Read the model definition and answer for the solid it produces. Units are mm, in the model's axes. Face numbers are marked on the shaded views. A direction names the side the tool comes from. Coordinates: 2 decimals unless noted, no trailing zeros. Loops run counter-clockwise (first coordinate to the right, second up) from the corner with the lowest first, then second, coordinate; pieces in that order, holes last. Notation, with made-up numbers: M 31,3.5 L 61,3.5 A17 cw 61,8.5 Z; hole C 43.5,34 d1. An arc over 180 degrees is marked long. One line per item, written item: value. Start each with the question number.
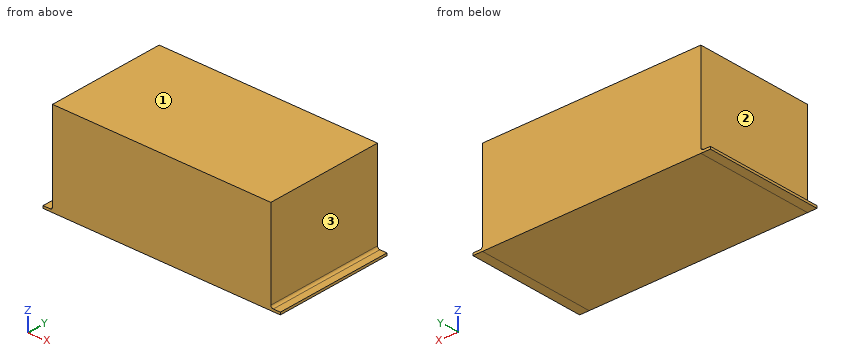
```python
from build123d import *

# Parameters (mm, degrees)
IZIM1_W                     = 920
IZIM1_H                     = 500
Y_KSEKLIK_EKSTR_ZYON1_DEPTH = 380
BO_ALTMA1_T                 = -0.6
IZIM2_W                     = 920
IZIM2_H                     = 500
Y_KSEKLIK_EKSTR_ZYON2_DEPTH = 1.8
IZIM3_W                     = 1000
IZIM3_H                     = 500
Y_KSEKLIK_EKSTR_ZYON3_DEPTH = 10
RADYUS1_R                   = 10
IZIM4_W                     = 918.8
IZIM4_H                     = 498.8
KES_EKSTR_ZYON1_DEPTH       = 5
RADYUS2_R                   = 20
IZIM5_W                     = 920
IZIM5_H                     = 500
KES_EKSTR_ZYON2_DEPTH       = 0.0001


with BuildPart() as part:
    # Çizim1 → Yükseklik-Ekstrüzyon1 (new body)
    with BuildSketch(Plane.XY):
        with Locations((460, 250)):
            Rectangle(IZIM1_W, IZIM1_H)
    extrude(amount=Y_KSEKLIK_EKSTR_ZYON1_DEPTH)

    # İç Boşaltma1
    bo_altma1_openings = [part.faces().sort_by_distance(p)[0] for p in [
        (460, 250, 380),
    ]]
    offset(amount=BO_ALTMA1_T, openings=bo_altma1_openings, kind=Kind.INTERSECTION)

    # Çizim2 → Yükseklik-Ekstrüzyon2 (add)
    with BuildSketch(Plane.XY.offset(380)):
        with Locations((460, 250)):
            Rectangle(IZIM2_W, IZIM2_H)
    extrude(amount=Y_KSEKLIK_EKSTR_ZYON2_DEPTH)

    # Çizim3 → Yükseklik-Ekstrüzyon3 (add)
    with BuildSketch(Plane(origin=(0, 0, 0), x_dir=(-1, 0, 0), z_dir=(0, 0, -1))):
        with Locations((-460, 250)):
            Rectangle(IZIM3_W, IZIM3_H)
    extrude(amount=Y_KSEKLIK_EKSTR_ZYON3_DEPTH)

    # Radyus1
    radyus1_edges = [part.edges().sort_by_distance(p)[0] for p in [
        (0, 250, 0),
        (920, 250, 0),
    ]]
    fillet(radyus1_edges, radius=RADYUS1_R)

    # Çizim4 → Kes-Ekstrüzyon1 (cut)
    with BuildSketch(Plane.XY.offset(0.6)):
        with Locations((460, 250)):
            Rectangle(IZIM4_W, IZIM4_H)
    extrude(amount=-KES_EKSTR_ZYON1_DEPTH, mode=Mode.SUBTRACT)

    # Radyus2
    radyus2_edges = [part.edges().sort_by_distance(p)[0] for p in [
        (919.4, 250, -4.4),
        (460, 0.6, -4.4),
        (0.6, 250, -4.4),
        (460, 499.4, -4.4),
    ]]
    fillet(radyus2_edges, radius=RADYUS2_R)

    # Çizim5 → Kes-Ekstrüzyon2 (cut)
    with BuildSketch(Plane(origin=(0, 0, -10), x_dir=(-1, 0, 0), z_dir=(0, 0, -1))):
        with Locations((-460, 250)):
            Rectangle(IZIM5_W, IZIM5_H)
    extrude(amount=-KES_EKSTR_ZYON2_DEPTH, mode=Mode.SUBTRACT)


solid = part.part
```
1) Consider line 1 along Z through (x, y) = (570, 118); line 2 along X through (y, z) = (297, 96.5); line 3 along Z through (x, y) = (18, 471.5). Determine where each line is inside the solid, lowest interval first.
2) Flat-ended cylindrical pins translate along their axes: pin 1 (24 mm diameter, centred on x = 939.5, y = 189, fed in from +Z); pin 2 (1.5 mm diameter, centred on y = 126.5, z = 280, fed in from -X); pin 3 (4 mm diameter, centred on y = 177, z = 281, fed in from +X). Find the tip coordinate at first contact, or state that the pin passes through.
3) Section C-C (z = 163) is taken. Determine the outline of the cut face in (x, y).
4) A tool of negligible diameter and unlimited length cuts with its end or side. For the marked faces 1, 2 and 3, from which of +Z, -Z, +X, -X, +Y, -Y can it reach the whole face along a straight path? Write none if from no direction.
Results found:
1. line 1: z = -10 to -4.4, 380 to 381.8
1. line 2: x = 0 to 0.6, 919.4 to 920
1. line 3: z = -10 to -4.23, 380 to 381.8
2. pin 1: stops at z = 0.32
2. pin 2: stops at x = 0
2. pin 3: stops at x = 920
3. outline: M 0,0 L 920,0 L 920,500 L 0,500 Z; hole M 0.6,0.6 L 919.4,0.6 L 919.4,499.4 L 0.6,499.4 Z
4. face 1: +Z, +X, -X, +Y, -Y
4. face 2: +Z, -X, +Y, -Y
4. face 3: +Z, +X, +Y, -Y
